The listing builds one solid part. Answer for the finished solid, in the listing's coordinates (mm). A direction names the side the tool comes from. Round coordinates to 2 decimals unless told otherwise and drop trailing zeros. Write each loop counter-clockwise with the first axis right and the second up, starting at its lowest first coordinate (ties: lowest second). Pieces come first, ordered by that corner, then holes.
Item 1: Find section B-B on y = 2.75. Give the vertices of the cut face in (x, z).
Item 2: Find section C-C on y = 10.75. Give the vertices of the cut face in (x, z), then the cut area to 3 significant figures.
Item 3: Find the intervals of material crossed by probe 1 along X at (y, z) = (9.65, 0); probe 2 along X at (y, z) = (2, 6); probe 3 along X at (y, z) = (8.7, -8.5), in increasing order.
Item 4: Each of these flat-tipped pins is pushed along its axis until it touches: pin 1 (4 mm diameter, centred on x = -7.36, z = 4.25, fed in from -Y); pin 2 (10 mm diameter, centred on x = 0, z = 0, fed in from -Y); pin 3 (1.5 mm diameter, centred on y = 7, z = -10, fed in from +X); pin 4 (3.5 mm diameter, centred on x = -1.5, z = -8, fed in from +Y). Where does it stop, or does it pass through?
Item 5: Find section A-A on x = 0. Give the vertices of the cut face in (y, z), then the cut area to 3 significant figures.
Item 6: A tool of negligible diameter and unlimited length cuts with its end or side. For faces 3 (the face through (0, 0, 7)), 4 (the face through (4.995, 3.752, 4.777)), 5 (the face through (-9, 8, 6)), from which of +Z, -Z, +X, -X, +Y, -Y can it reach the whole face along a straight path? Write none if from no direction.
Item 7: For a pull along Z with two mould halves and no side action, classify faces 1 (the face through (4, 12, -4)), 2 (the face through (-9.224, 4.056, 5.219)) as +Z half, -Z half, draft (parallel to the pull), parting line (faces both ways), or undercut.
```python
from build123d import *

# Parameters (mm, degrees)
SKETCH1_R           = 15.5
BOSS_EXTRUDE1_DEPTH = 12
SKETCH2_R           = 2.1
CUT_EXTRUDE1_DEPTH  = 25.989997999
SKETCH3_R           = 4.25
CUT_EXTRUDE2_DEPTH  = 25.989997999
CUT_EXTRUDE3_DEPTH  = 7.4
SKETCH5_R           = 3.65
CUT_EXTRUDE4_DEPTH  = 4
CHAMFER1_SIZE       = 0.5
FILLET_1_R          = 0.5


with BuildPart() as part:
    # Sketch1 → Boss-Extrude1 (new body)
    with BuildSketch(Plane(origin=(0, 0, 0), x_dir=(1, 0, 0), z_dir=(0, 1, 0))):
        with Locations(Location((0, 0, 0), (0, 0, 270))):
            Circle(SKETCH1_R)
    extrude(amount=BOSS_EXTRUDE1_DEPTH)

    # Sketch2 → Cut-Extrude1 (cut, through all)
    with BuildSketch(Plane(origin=(0, 12, 0), x_dir=(1, 0, 0), z_dir=(0, 1, 0))):
        with Locations(Location((0, 8.5, 0), (0, 0, 270))):
            Circle(SKETCH2_R)
        with Locations(Location((7.361215932, -4.25, 0), (0, 0, 270))):
            Circle(SKETCH2_R)
        with Locations(Location((-7.361215932, -4.25, 0), (0, 0, 270))):
            Circle(SKETCH2_R)
    extrude(amount=-CUT_EXTRUDE1_DEPTH, mode=Mode.SUBTRACT)

    # Sketch3 → Cut-Extrude2 (cut, through all)
    with BuildSketch(Plane(origin=(0, 12, 0), x_dir=(1, 0, 0), z_dir=(0, 1, 0))):
        with Locations(Location((0, 0, 0), (0, 0, 270))):
            Circle(SKETCH3_R)
    extrude(amount=-CUT_EXTRUDE2_DEPTH, mode=Mode.SUBTRACT)

    # Sketch4 → Cut-Extrude3 (cut)
    with BuildSketch(Plane.XZ):
        Polygon((3.740942098, -6.44013604), (7.447792464, 0.019682871), (3.706850366, 6.459818911), (-3.740942098, 6.44013604), (-7.447792464, -0.019682871), (-3.706850366, -6.459818911), align=None)
    extrude(amount=-CUT_EXTRUDE3_DEPTH, mode=Mode.SUBTRACT)

    # Sketch5 → Cut-Extrude4 (cut)
    with BuildSketch(Plane(origin=(0, 12, 0), x_dir=(1, 0, 0), z_dir=(0, 1, 0))):
        with Locations(Location((0, 8.5, 0), (0, 0, 270))):
            Circle(SKETCH5_R)
        with Locations(Location((7.361215932, -4.25, 0), (0, 0, 270))):
            Circle(SKETCH5_R)
        with Locations(Location((-7.361215932, -4.25, 0), (0, 0, 270))):
            Circle(SKETCH5_R)
    extrude(amount=-CUT_EXTRUDE4_DEPTH, mode=Mode.SUBTRACT)

    # Chamfer1
    # the kernel refuses this chamfer: 0.5 mm, written as the material it takes off along each edge
    with BuildSketch(Plane(origin=(0, 12, 0), x_dir=(0, 0, 1), z_dir=(-1, 0, 0))) as chamfer1_piece_1:
        Polygon((4.25 + CHAMFER1_SIZE, 0), (4.25, -CHAMFER1_SIZE), (4.25, 0), align=None)
    revolve(axis=Axis((0, 12, 0), (0, 1, 0)), mode=Mode.SUBTRACT)
    with BuildSketch(Plane(origin=(0, 12, 0), x_dir=(0, 0, 1), z_dir=(-1, 0, 0))) as chamfer1_piece_2:
        Polygon((15.5, -CHAMFER1_SIZE), (15.5 - CHAMFER1_SIZE, 0), (15.5, 0), align=None)
    revolve(axis=Axis((0, 12, 0), (0, 1, 0)), mode=Mode.SUBTRACT)
    with BuildSketch(Plane(origin=(0, 12, -8.5), x_dir=(0, 0, 1), z_dir=(-1, 0, 0))) as chamfer1_piece_3:
        Polygon((3.65 + CHAMFER1_SIZE, 0), (3.65, -CHAMFER1_SIZE), (3.65, 0), align=None)
    revolve(axis=Axis((0, 12, -8.5), (0, 1, 0)), mode=Mode.SUBTRACT)
    with BuildSketch(Plane(origin=(7.361215932, 12, 4.25), x_dir=(0, 0, 1), z_dir=(-1, 0, 0))) as chamfer1_piece_4:
        Polygon((3.65 + CHAMFER1_SIZE, 0), (3.65, -CHAMFER1_SIZE), (3.65, 0), align=None)
    revolve(axis=Axis((7.361215932, 12, 4.25), (0, 1, 0)), mode=Mode.SUBTRACT)
    with BuildSketch(Plane(origin=(-7.361215932, 12, 4.25), x_dir=(0, 0, 1), z_dir=(-1, 0, 0))) as chamfer1_piece_5:
        Polygon((3.65 + CHAMFER1_SIZE, 0), (3.65, -CHAMFER1_SIZE), (3.65, 0), align=None)
    revolve(axis=Axis((-7.361215932, 12, 4.25), (0, 1, 0)), mode=Mode.SUBTRACT)

    # Скругление1
    fillet_1_edges = [part.edges().sort_by_distance(p)[0] for p in [
        (5.359734874, 3.7, 3.614332183),
        (5.817474247, 3.7, 2.826321101),
        (-5.809970925, 3.7, 2.834500467),
        (-5.356402996, 3.7, 3.624919933),
        (0.450236051, 3.7, -6.44883265),
        (-0.461071251, 3.7, -6.451241034),
    ]]
    fillet(fillet_1_edges, radius=FILLET_1_R)


solid = part.part
```
Check values:
1. outline: circle Ø31 at (0, 0); hole (-7.45, -0.02) - (-3.71, -6.46) - (-2.09, -6.46) arc R0.5 cw to (-1.69, -7.25) arc R2.1 ccw (long way) to (1.68, -7.24) arc R0.5 cw to (2.08, -6.44) - (3.74, -6.44) - (7.45, 0.02) - (6.64, 1.42) arc R0.5 cw to (7.13, 2.16) arc R2.1 ccw (long way) to (5.43, 5.08) arc R0.5 cw to (4.54, 5.03) - (3.71, 6.46) - (-3.74, 6.44) - (-4.54, 5.04) arc R0.5 cw to (-5.44, 5.09) arc R2.1 ccw (long way) to (-7.11, 2.16) arc R0.5 cw to (-6.62, 1.42) - close
2. outline: circle Ø31 at (0, 0); hole circle Ø7.3 at (-7.36, 4.25); hole circle Ø8.5 at (0, 0); hole circle Ø7.3 at (0, -8.5); hole circle Ø7.3 at (7.36, 4.25)
2. area: 572 mm2
3. probe 1: x = -15.5 to -4.25, 4.25 to 15.5
3. probe 2: x = -14.29 to -8.52, -6.2 to -3.99, 3.97 to 6.2, 8.52 to 14.29
3. probe 3: x = -12.96 to -3.65, 3.65 to 12.96
4. pin 1: passes through
4. pin 2: stops at y = 7.4
4. pin 3: stops at x = 12.44
4. pin 4: stops at y = 8
5. outline: (0, -15.5) - (11.5, -15.5) - (12, -15) - (12, -12.65) - (11.5, -12.15) - (8, -12.15) - (8, -10.6) - (0, -10.6) - close; (0, 6.45) - (7.4, 6.45) - (7.4, 4.25) - (11.5, 4.25) - (12, 4.75) - (12, 15) - (11.5, 15.5) - (0, 15.5) - close; (7.4, -6.4) - (8, -6.4) - (8, -4.85) - (11.5, -4.85) - (11.8, -4.55) - (11.5, -4.25) - (7.4, -4.25) - close
5. area: 174 mm2
6. face 3: +Z, -Z, +X, -X, -Y
6. face 4: -Y
6. face 5: +Y
7. face 1: draft
7. face 2: undercut
